CAD build for the part. Positions are in the model's coordinates, mm. Face numbers are marked on the shaded views. A direction names the side the tool comes from. Coordinates: 2 decimals unless noted, no trailing zeros. Loops run counter-clockwise (first coordinate to the right, second up) from the corner with the lowest first, then second, coordinate; pieces in that order, holes last.
1) Saw through at C-C, the plane y = 46. Write the cut outline in (x, z), and give its area (3 significant figures).
2) Saw through at A-A, the plane y = 5.5. Write the cut outline in (x, z).
3) Wall check: line 1 along Y through (x, z) = (-40, -8); line 2 along Y through (x, z) = (-20, -2); line 3 along X through (y, z) = (29, -6.25). Give the ranges that are in metal, low to high.
4) Which spindle directions (+Z, -Z, +X, -X, +Y, -Y) get a long thin tool onto all of the face, cutting with end or side? Do the marked faces 1 and 2. Say none if no direction does.
5) Saw through at B-B, the plane x = -31.5. Write the cut outline in (y, z).
6) Pin check, flat tips, straight feed: pin 1 Ø1.5 at (x, y) = (40, 5.5) entering from +Z; pin 2 Ø0.9 at (y, z) = (5, -1) entering from +X; pin 3 Ø1.6 at (y, z) = (54, -5) entering from -X. Stop position of each tip, or through.
```python
from build123d import *

# Parameters (mm, degrees)
ESQUISSE1_W             = 145
ESQUISSE1_H             = 10
BOSS_EXTRU_1_DEPTH      = 11
ESQUISSE2_R             = 1.5
ENL_V_MAT_EXTRU_1_DEPTH = 75.008445464
ESQUISSE3_R             = 1.5
ENL_V_MAT_EXTRU_2_DEPTH = 75.008445464
ENL_V_MAT_EXTRU_3_DEPTH = 3
ENL_V_MAT_EXTRU_4_DEPTH = 3
CONG_1_R                = 9
ESQUISSE6_W             = 8
ESQUISSE6_H             = 10
BOSS_EXTRU_2_DEPTH      = 49.5
CONG_2_R                = 3
ESQUISSE7_R             = 1.5
ENL_V_MAT_EXTRU_5_DEPTH = 158.433319218
ENL_V_MAT_EXTRU_6_DEPTH = 3
BOSS_EXTRU_3_START      = -0.2
BOSS_EXTRU_3_DEPTH      = 0.2


with BuildPart() as part:
    # Esquisse1 → Boss.-Extru.1 (new body)
    with BuildSketch(Plane(origin=(0, 0, 0), x_dir=(1, 0, 0), z_dir=(0, 1, 0))):
        with Locations((0, 5)):
            Rectangle(ESQUISSE1_W, ESQUISSE1_H)
    extrude(amount=BOSS_EXTRU_1_DEPTH)

    # Esquisse2 → Enlèv. mat.-Extru.1 (cut, through all)
    with BuildSketch(Plane(origin=(0, 11, 0), x_dir=(1, 0, 0), z_dir=(0, 1, 0))):
        with Locations(Location((-57.5, 4, 0), (0, 0, 270))):
            Circle(ESQUISSE2_R)
        with Locations(Location((57.5, 4, 0), (0, 0, 270))):
            Circle(ESQUISSE2_R)
    extrude(amount=-ENL_V_MAT_EXTRU_1_DEPTH, mode=Mode.SUBTRACT)

    # Esquisse3 → Enlèv. mat.-Extru.2 (cut, through all)
    with BuildSketch(Plane.XY):
        with Locations((-40, 5.5)):
            Circle(ESQUISSE3_R)
        with Locations(Location((40, 5.5, 0), (0, 0, 180))):
            Circle(ESQUISSE3_R)
    extrude(amount=-ENL_V_MAT_EXTRU_2_DEPTH, mode=Mode.SUBTRACT)

    # Esquisse4 → Enlèv. mat.-Extru.3 (cut)
    with BuildSketch(Plane.XY):
        Polygon((-37.25, 7.08771324), (-40, 8.675426481), (-42.75, 7.08771324), (-42.75, 3.91228676), (-40, 2.324573519), (-37.25, 3.91228676), align=None)
        Polygon((42.75, 7.08771324), (40, 8.675426481), (37.25, 7.08771324), (37.25, 3.91228676), (40, 2.324573519), (42.75, 3.91228676), align=None)
    extrude(amount=-ENL_V_MAT_EXTRU_3_DEPTH, mode=Mode.SUBTRACT)

    # Esquisse5 → Enlèv. mat.-Extru.4 (cut)
    with BuildSketch(Plane(origin=(0, 11, 0), x_dir=(1, 0, 0), z_dir=(0, 1, 0))):
        Polygon((-54.75, 5.58771324), (-57.5, 7.175426481), (-60.25, 5.58771324), (-60.25, 2.41228676), (-57.5, 0.824573519), (-54.75, 2.41228676), align=None)
        Polygon((60.25, 5.58771324), (57.5, 7.175426481), (54.75, 5.58771324), (54.75, 2.41228676), (57.5, 0.824573519), (60.25, 2.41228676), align=None)
    extrude(amount=-ENL_V_MAT_EXTRU_4_DEPTH, mode=Mode.SUBTRACT)

    # Congé1
    cong_1_edges = [part.edges().sort_by_distance(p)[0] for p in [
        (72.5, 0, -5),
    ]]
    fillet(cong_1_edges, radius=CONG_1_R)

    # Esquisse6 → Boss.-Extru.2 (add)
    with BuildSketch(Plane(origin=(0, 11, 0), x_dir=(1, 0, 0), z_dir=(0, 1, 0))):
        with Locations((68.5, 5)):
            Rectangle(ESQUISSE6_W, ESQUISSE6_H)
    extrude(amount=BOSS_EXTRU_2_DEPTH)

    # Congé2
    cong_2_edges = [part.edges().sort_by_distance(p)[0] for p in [
        (64.5, 11, -5),
    ]]
    fillet(cong_2_edges, radius=CONG_2_R)

    # Esquisse7 → Enlèv. mat.-Extru.5 (cut, through all)
    with BuildSketch(Plane(origin=(72.5, 0, 0), x_dir=(0, 0, -1), z_dir=(1, 0, 0))):
        with Locations((4, 54.5)):
            Circle(ESQUISSE7_R)
    extrude(amount=-ENL_V_MAT_EXTRU_5_DEPTH, mode=Mode.SUBTRACT)

    # Esquisse8 → Enlèv. mat.-Extru.6 (cut)
    with BuildSketch(Plane.ZY.offset(-64.5)):
        Polygon((-0.824573519, 54.5), (-2.41228676, 57.25), (-5.58771324, 57.25), (-7.175426481, 54.5), (-5.58771324, 51.75), (-2.41228676, 51.75), align=None)
    extrude(amount=-ENL_V_MAT_EXTRU_6_DEPTH, mode=Mode.SUBTRACT)

    # Esquisse9 → Boss.-Extru.3 (add)
    with BuildSketch(Plane(origin=(0, 0, -10), x_dir=(-1, 0, 0), z_dir=(0, 0, -1)).offset(BOSS_EXTRU_3_START)):
        with BuildLine():
            Line((-72.5, 60.5), (-72.5, 9))
            ThreePointArc((-72.5, 9), (-69.863961031, 2.636038969), (-63.5, 0))
            Line((-63.5, 0), (72.5, 0))
            Line((72.5, 0), (72.5, 11))
            Line((72.5, 11), (-61.5, 11))
            ThreePointArc((-61.5, 11), (-63.621320344, 11.878679656), (-64.5, 14))
            Line((-64.5, 14), (-64.5, 60.5))
            Line((-64.5, 60.5), (-72.5, 60.5))
        make_face()
    extrude(amount=BOSS_EXTRU_3_DEPTH)


solid = part.part
```
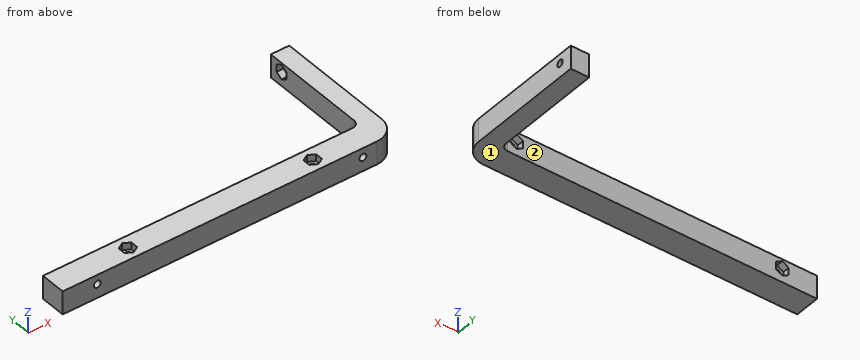
Data:
1. outline: (64.5, -10) - (72.5, -10) - (72.5, 0) - (64.5, 0) - close
1. area: 80.0 mm2
2. outline: (-72.5, -10) - (71.79, -10) - (71.79, 0) - (42.75, 0) - (42.75, -3) - (41.5, -3) - (41.5, -9.8) - (38.5, -9.8) - (38.5, -3) - (37.25, -3) - (37.25, 0) - (-37.25, 0) - (-37.25, -3) - (-38.5, -3) - (-38.5, -9.8) - (-41.5, -9.8) - (-41.5, -3) - (-42.75, -3) - (-42.75, 0) - (-72.5, 0) - close; hole circle Ø3 at (-57.5, -4); hole circle Ø3 at (57.5, -4)
3. line 1: y = 0 to 4, 7 to 11
3. line 2: y = 0 to 11
3. line 3: x = 64.5 to 72.5
4. face 1: -Z, +X, -X, +Y, -Y
4. face 2: +Z, -Z, -X, +Y
5. outline: (0, -10) - (11, -10) - (11, 0) - (0, 0) - close
6. pin 1: stops at z = -9.8
6. pin 2: stops at x = 71.77
6. pin 3: stops at x = 67.5
